Autodesk Inventor part; units mm, degrees
ref_plane "YZ Plane" through (0, 0, 0) normal (1, 0, 0) x (0, 1, 0)
ref_plane "XZ Plane" through (0, 0, 0) normal (0, 1, 0) x (-1, 0, 0)
ref_plane "XY Plane" through (0, 0, 0) normal (0, 0, 1) x (1, 0, 0)
sketch "Sketch1" plane through (0, 0, 0) normal (0, 0, 1) x (1, 0, 0)
  line L0 (-46, -50) -> (46, -50)
  line L1 (46, -50) -> (46, 50)
  line L2 (46, 50) -> (-46, 50)
  line L3 (-46, 50) -> (-46, -50)
  line L4 (-46, -50) -> (46, 50) construction
  line L5 (46, -50) -> (-46, 50) construction
  point P0 (0, 0)
  dimension "d154" = 92
  dimension "d155" = 100
extrude "Plate5" add sketch "Sketch1" along normal blind 2
sketch "Sketch7" plane through (-44, -50, 0) normal (-1, 0, 0) x (0, -1, 0)
  line L0 (-100, 0) -> (0, 0)
  line L1 (0, 0) -> (0, 94)
  line L2 (0, 94) -> (-100, 94)
  line L3 (-100, 94) -> (-100, 0)
edge flange "Flange3" height 94 angle 90 thickness 2 bend radius 2.75 thickness toward (-1, 0, 0) relief round relief width 2 relief depth 1 edges at (-46, 0, 2) wall of the first edge with corners at (-44, 50, 0) (-44, -50, 0) (-44, -50, 94) (-44, 50, 94)
bend "Bend3"
corner "Corner3"
sketch "Sketch8" plane through (0, 0, 2) normal (0, 0, 1) x (1, 0, 0)
  line L0 (46, 50) -> (46, -50)
  line L1 (-41.25, 50) -> (46, 50)
  line L2 (29, 45) -> (-27, 45)
  line L3 (-27, 45) -> (-27, -11)
  line L4 (-27, -11) -> (29, -11)
  line L5 (29, -11) -> (29, 45)
  line L6 (29, 45) -> (-27, -11) construction
  line L7 (-27, 45) -> (29, -11) construction
  point P0 (0, 0)
  point P1 (1, 17)
  point P2 (2.375, 50)
  dimension "d167" = 56
  dimension "d168" = 56
  dimension "d169" = 5
  dimension "d172" = 17
extrude "Cut1" cut sketch "Sketch8" against normal blind 2
properties part number "TZS 752 FDS 1200 FLANGE 2" material "Stainless Steel"
Here's how the part is built. I have some questions about the finished solid (model axes, mm). A direction names the side the tool comes from. Round coordinates to 2 decimals unless told otherwise and drop trailing zeros. Loops run counter-clockwise (first coordinate to the right, second up) from the corner with the lowest first, then second, coordinate; pieces in that order, holes last.
1. If I drill on line 1 along Z through (x, y) = (-34.5, -4); line 2 along X through (y, z) = (-3.5, 59), over which ranges is the centre line in solid material (lowest first)?
Answer list:
line 1: z = 0 to 2
line 2: x = -46 to -44
2. Which directions (+Z, -Z, +X, -X, +Y, -Y) give clear straight access to the entire face, cutting with the end or side of a thin tool? Please do faces 1 (the face through (-46, -1, 50)), 2 (the face through (2, -22, 2)).
Answer list:
face 1: +Z, -Z, -X, +Y, -Y
face 2: +Z, +X, +Y, -Y
3. If we section it at D-D on z = 17.5: Write out the boundary of the cut face in (x, y).
Answer list:
outline: (-46, -50) - (-44, -50) - (-44, 50) - (-46, 50) - close
4. For P1, Ø2, axis at y = 17.5, z = 70, coming from the +X side; P2, Ø10, axis at x = -17.5, y = 14.5, coming from the -Z side; P3, Ø2, axis at y = 21, z = 0.5, coming from the -X side, each with a flat end and sliding along its axis, tell me the tip position at first contact or that it passes through.
Answer list:
P1: stops at x = -44
P2: passes through
P3: stops at x = -44.71
5. If we section it at B-B on y = 14: Write out the boundary of the cut face in (x, z), plus the area to 3 significant figures.
Answer list:
outline: (-46, 4.75) arc R4.75 ccw to (-41.25, 0) - (-27, 0) - (-27, 2) - (-41.25, 2) arc R2.75 cw to (-44, 4.75) - (-44, 94) - (-46, 94) - close; (29, 0) - (46, 0) - (46, 2) - (29, 2) - close
area: 253 mm2
6. If we section it at A-A on x = 26.5: Write out the boundary of the cut face in (y, z), plus the area to 3 significant figures.
Answer list:
outline: (-50, 0) - (-11, 0) - (-11, 2) - (-50, 2) - close; (45, 0) - (50, 0) - (50, 2) - (45, 2) - close
area: 88.0 mm2
7. If we section it at C-C on y = -21: Write out the boundary of the cut face in (x, z), plus the area to 3 significant figures.
Answer list:
outline: (-46, 4.75) arc R4.75 ccw to (-41.25, 0) - (46, 0) - (46, 2) - (-41.25, 2) arc R2.75 cw to (-44, 4.75) - (-44, 94) - (-46, 94) - close
area: 365 mm2
